The listing builds one solid part. Answer for the finished solid, in the listing's coordinates (mm). Face numbers are marked on the shaded views. A direction names the side the tool comes from. Give positions to 0.01 mm unless a question says otherwise; leave off trailing zeros. Order: outer loops, then holes, each group sorted by start corner. A loop starts at its lowest first (then second) coordinate and runs counter-clockwise, first axis right, second up. Notation, with made-up numbers: (57.25, 88.5) - (77.25, 88.5) arc R32 cw to (77.25, 123.5) - close; hole circle Ø3 at (53.25, -15). An arc over 180 degrees is marked (long way). Answer as a JSON object with one key per item and string values. Group by question number.
Q1. Given pin 1 (1.5 mm diameter, centred on y = -38, z = 1, fed in from +X); pin 2 (1.3 mm diameter, centred on x = -10, z = 0, fed in from +Y); pin 3 (1.5 mm diameter, centred on x = -9, y = -45.5, fed in from +Z), each flat-ended and moving along its own axis, determine where each tip first touches the part or whether it passes through.
Q2. For the marked faces 1 and 2, determine the directions among +Z, -Z, +X, -X, +Y, -Y from which every point of the face is accessible in a straight line to the end or side of a thin tool.
Q3. A cutting plane is placed at B-B, the plane z = 0. Give the vertices of the cut face in (x, y), and give its area (3 significant figures).
Q4. Consider line 1 (Y direction, x = -9.5, z = 0.25); line 2 (Z direction, x = -9.25, y = -44.25); line 3 (Z direction, x = -8.25, y = -32.5). Determine where each line is inside the solid, lowest interval first.
Q5. A cutting plane is placed at A-A, the plane y = -34. Give the vertices of the cut face in (x, z), and give its area (3 significant figures).
Q6. The mould has two halves that part along Z. Classify the marked faces 3, 4 and 5: released by +Z, released by -Z, zero draft, split by the parting line, or undercut.
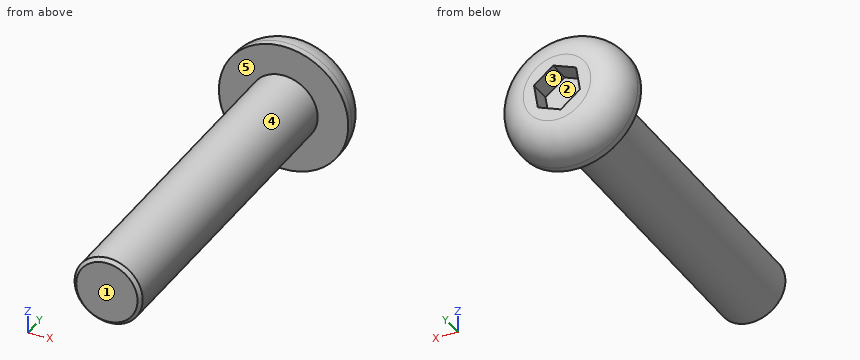
Autodesk Inventor part; units mm, degrees
ref_plane "YZ Plane" through (0, 0, 0) normal (1, 0, 0) x (0, 1, 0)
ref_plane "XZ Plane" through (0, 0, 0) normal (0, 1, 0) x (-1, 0, 0)
ref_plane "XY Plane" through (0, 0, 0) normal (0, 0, 1) x (1, 0, 0)
sketch "Sketch1" plane through (0, 0, 0) normal (0, 0, 1) x (1, 0, 0)
  line L0 (-9.677, -30.5907) -> (-13.477, -30.5907)
  line L1 (-9.677, -30.5907) -> (-9.677, -50.5907)
  line L2 (-9.677, -50.5907) -> (-11.677, -50.5907)
  line L3 (-11.677, -50.5907) -> (-11.677, -30.5907)
  line L4 (-9.677, -30.5907) -> (-9.677, -26.5988)
  line L5 (-13.477, -30.5907) -> (-13.477, -30.2107)
  line L6 (-13.477, -30.2107) -> (-13.477, -28.3907)
  line L7 (-13.477, -28.3907) -> (-9.677, -28.3907)
  point P0 (0, 0)
  dimension "d0" = 3.8
  dimension "d2" = 20
  dimension "d3" = 2
  dimension "d18" = 0.38
  dimension "d19" = 2.2
revolve "Revolution1" add sketch "Sketch1" angle 360 about axis through (-9.677, -30.5907, 0) along (0, -1, 0)
chamfer "Chamfer2" distance 0.2 angle 45 1 edges at (-7.677, -50.5907, 0)
thread "Rosca1"
fillet "Empalme2" radius 1.82 1 edges at (-5.877, -28.3907, 0)
sketch "Boceto2" plane through (-9.677, -28.3907, 0) normal (0, 1, 0) x (1, 0, 0)
  line L0 (1.1232, 0.9065) -> (1.3467, -0.5194)
  line L1 (1.3467, -0.5194) -> (0.2235, -1.426)
  line L2 (0.2235, -1.426) -> (-1.1232, -0.9065)
  line L3 (-1.1232, -0.9065) -> (-1.3467, 0.5194)
  line L4 (-1.3467, 0.5194) -> (-0.2235, 1.426)
  line L5 (-0.2235, 1.426) -> (1.1232, 0.9065)
  point P0 (9.677, 0)
  point P1 (0, 0)
  dimension "d21" = 2.5
extrude "Extrusión1" cut sketch "Boceto2" against normal blind 1.3
properties part number "Tornillo Allen cabeza botón M4x20mm"
Reply:
{
 "1": {"pin 1": "stops at x = -7.69", "pin 2": "stops at y = -29.69", "pin 3": "stops at z = 2"},
 "2": {"face 1": "+Z, -Z, +X, -X, -Y", "face 2": "+Y"},
 "3": {"outline": "(-13.48, -30.59) - (-11.68, -30.59) - (-11.68, -50.39) - (-11.48, -50.59) - (-7.88, -50.59) - (-7.68, -50.39) - (-7.68, -30.59) - (-5.88, -30.59) - (-5.88, -30.21) arc R1.82 ccw to (-7.7, -28.39) - (-8.41, -28.39) - (-8.41, -29.69) - (-10.94, -29.69) - (-10.94, -28.39) - (-11.66, -28.39) arc R1.82 ccw to (-13.48, -30.21) - close", "area": "92.0 mm^2"},
 "4": {"line 1": "y = -50.59 to -29.69", "line 2": "z = -1.95 to 1.95", "line 3": "z = -1.4 to 1.4"},
 "5": {"outline": "circle Ø4 at (-9.68, 0)", "area": "12.6 mm^2"},
 "6": {"face 3": "undercut", "face 4": "split by the parting line", "face 5": "zero draft"}
}
